```python
from build123d import *

# Parameters (mm, degrees)
SKETCH_1_W          = 70
SKETCH_1_H          = 50
EXTRUDE_1_DEPTH     = 1.6
CUT_EXTRUDE_1_REACH = 45.041
SKETCH_2_R          = 1.65
SKETCH_3_W          = 70
SKETCH_3_H          = 12.5
EXTRUDE_2_DEPTH     = 1.6
CHAMFER_1_SIZE      = 3


with BuildPart() as part:
    # 草图1 → 凸台-拉伸1 (new body)
    with BuildSketch(Plane(origin=(0, 0, 0), x_dir=(1, 0, 0), z_dir=(0, 1, 0))):
        Rectangle(SKETCH_1_W, SKETCH_1_H)
    extrude(amount=EXTRUDE_1_DEPTH)

    # 草图2 → 切除-拉伸1 (cut, up to next)
    with BuildSketch(Plane(origin=(0, 1.6, 0), x_dir=(1, 0, 0), z_dir=(0, 1, 0)), mode=Mode.PRIVATE) as cut_extrude_1_sk1:
        with Locations(Location((-28, 20, 0), (0, 0, 270))):
            Circle(SKETCH_2_R)
    cut_extrude_1_tool1 = extrude(cut_extrude_1_sk1.sketch, amount=-CUT_EXTRUDE_1_REACH, mode=Mode.PRIVATE) & part.part
    # 草图2 → 切除-拉伸1 (cut, up to next)
    with BuildSketch(Plane(origin=(0, 1.6, 0), x_dir=(1, 0, 0), z_dir=(0, 1, 0)), mode=Mode.PRIVATE) as cut_extrude_1_sk2:
        with Locations(Location((-28, -20, 0), (0, 0, 270))):
            Circle(SKETCH_2_R)
    cut_extrude_1_tool2 = extrude(cut_extrude_1_sk2.sketch, amount=-CUT_EXTRUDE_1_REACH, mode=Mode.PRIVATE) & part.part
    # 草图2 → 切除-拉伸1 (cut, up to next)
    with BuildSketch(Plane(origin=(0, 1.6, 0), x_dir=(1, 0, 0), z_dir=(0, 1, 0)), mode=Mode.PRIVATE) as cut_extrude_1_sk3:
        with Locations(Location((28, -20, 0), (0, 0, 270))):
            Circle(SKETCH_2_R)
    cut_extrude_1_tool3 = extrude(cut_extrude_1_sk3.sketch, amount=-CUT_EXTRUDE_1_REACH, mode=Mode.PRIVATE) & part.part
    # 草图2 → 切除-拉伸1 (cut, up to next)
    with BuildSketch(Plane(origin=(0, 1.6, 0), x_dir=(1, 0, 0), z_dir=(0, 1, 0)), mode=Mode.PRIVATE) as cut_extrude_1_sk4:
        with Locations(Location((28, 20, 0), (0, 0, 270))):
            Circle(SKETCH_2_R)
    cut_extrude_1_tool4 = extrude(cut_extrude_1_sk4.sketch, amount=-CUT_EXTRUDE_1_REACH, mode=Mode.PRIVATE) & part.part
    add(cut_extrude_1_tool1.solids().sort_by_distance((-28, 1.6, -20))[0], mode=Mode.SUBTRACT)
    add(cut_extrude_1_tool2.solids().sort_by_distance((-28, 1.6, 20))[0], mode=Mode.SUBTRACT)
    add(cut_extrude_1_tool3.solids().sort_by_distance((28, 1.6, 20))[0], mode=Mode.SUBTRACT)
    add(cut_extrude_1_tool4.solids().sort_by_distance((28, 1.6, -20))[0], mode=Mode.SUBTRACT)

    # 草图3 → 凸台-拉伸2 (add)
    with BuildSketch(Plane(origin=(0, 0, 0), x_dir=(1, 0, 0), z_dir=(0, 1, 0))):
        Polygon((-35, -25), (-30, -30), (30, -30), (35, -25), align=None)
        with Locations((0, 31.25)):
            Rectangle(SKETCH_3_W, SKETCH_3_H)
    extrude(amount=EXTRUDE_2_DEPTH)

    # 倒角1
    chamfer_1_edges = [part.edges().sort_by_distance(p)[0] for p in [
        (35, 0.8, -37.5),
        (-35, 0.8, -37.5),
    ]]
    chamfer(chamfer_1_edges, length=CHAMFER_1_SIZE)


solid = part.part
```
Can you work these out from the model? Positions are in its coordinate system, mm. Coordinates: 2 decimals unless noted, no trailing zeros. Loops run counter-clockwise (first coordinate to the right, second up) from the corner with the lowest first, then second, coordinate; pieces in that order, holes last. Notation, with made-up numbers: M 32.25,54.5 L 53.25,54.5 A18 ccw 53.25,83.5 Z; hole C 60.25,3 d11. An arc over 180 degrees is marked long. Put each result on its own line as item: value. Start each with the question number.
(1) We'd pull the mould along Z, two halves only. Please class faces 1 (the face through (-26.364, 0.811, 19.785)), 2 (the face through (0, 0, -4)), 3 (the face through (32, 1, 28)), 4 (the face through (33.5, 0.8, -36)): +Z half, -Z half, draft (parallel to the pull), parting line (faces both ways), or undercut.
(2) Imagine slicing it at B-B on x = -28. List the corners of the cut face in (y, z) for me.
(3) Imagine slicing it at A-A on z = 20. List the corners of the cut face in (x, y) for me.
(4) I need wall thicknesses on probe 1 along X at (y, z) = (1.25, -20); probe 2 along X at (y, z) = (0.5, 26.5). Which ranges of each line are inside material? Lowest first, please.
Worked answers:
1. face 1: undercut
1. face 2: draft
1. face 3: +Z half
1. face 4: -Z half
2. outline: M 0,-37.5 L 1.6,-37.5 L 1.6,-21.65 L 0,-21.65 Z; M 0,-18.35 L 1.6,-18.35 L 1.6,18.35 L 0,18.35 Z; M 0,21.65 L 1.6,21.65 L 1.6,30 L 0,30 Z
3. outline: M -35,0 L -29.65,0 L -29.65,1.6 L -35,1.6 Z; M -26.35,0 L 26.35,0 L 26.35,1.6 L -26.35,1.6 Z; M 29.65,0 L 35,0 L 35,1.6 L 29.65,1.6 Z
4. probe 1: x = -35 to -29.65, -26.35 to 26.35, 29.65 to 35
4. probe 2: x = -33.5 to 33.5
